from build123d import *

# Parameters (mm, degrees)
BOSS_EXTRUDE1_DEPTH      = 100
BOSS_EXTRUDE1_DEPTH_BACK = 12.5
SKETCH1_W                = 25
SKETCH1_H                = 20
SKETCH2_W                = 15
SKETCH2_H                = 10
CUT_EXTRUDE1_DEPTH       = 103.74361294
CUT_EXTRUDE2_DEPTH       = 103.74361294


with BuildPart() as part:
    # Sketch1 → Boss-Extrude1 (new, two sides: drawn at the far end of the back side and taken through both)
    with BuildSketch(Plane(origin=(0, 0, 0), x_dir=(1, 0, 0), z_dir=(0, 1, 0)).offset(-BOSS_EXTRUDE1_DEPTH_BACK)):
        Rectangle(SKETCH1_W, SKETCH1_H)
    extrude(amount=BOSS_EXTRUDE1_DEPTH + BOSS_EXTRUDE1_DEPTH_BACK)

    # Sketch2 → Cut-Extrude1 (cut, through all)
    with BuildSketch(Plane.XY.offset(10)):
        with Locations((0, 91.5)):
            Rectangle(SKETCH2_W, SKETCH2_H)
    extrude(amount=-CUT_EXTRUDE1_DEPTH, mode=Mode.SUBTRACT)

    # Sketch3 → Cut-Extrude2 (cut, through all)
    with BuildSketch(Plane.XY.offset(10)):
        with BuildLine():
            Line((-3.5, -2.5), (3.5, -2.5))
            ThreePointArc((3.5, -2.5), (7.035533906, -1.035533906), (8.5, 2.5))
            Line((8.5, 2.5), (8.5, 70))
            ThreePointArc((8.5, 70), (7.035533906, 73.535533906), (3.5, 75))
            Line((3.5, 75), (-3.5, 75))
            ThreePointArc((-3.5, 75), (-7.035533906, 73.535533906), (-8.5, 70))
            Line((-8.5, 70), (-8.5, 2.5))
            ThreePointArc((-8.5, 2.5), (-7.035533906, -1.035533906), (-3.5, -2.5))
        make_face()
    extrude(amount=-CUT_EXTRUDE2_DEPTH, mode=Mode.SUBTRACT)


solid = part.part
Work out the finished part from the listing and answer in its coordinate system (mm). A direction names the side the tool comes from. Round coordinates to 2 decimals unless told otherwise and drop trailing zeros. Write each loop counter-clockwise with the first axis right and the second up, starting at its lowest first coordinate (ties: lowest second). Pieces come first, ordered by that corner, then holes.
1) A cutting plane is placed at A-A (y = 16). Give the vertices of the cut face in (x, z).
2) Straight lines are drawn through the part: line 1 (Y direction, x = 2, z = -9); line 2 (X direction, y = 6.5, z = 8.75); line 3 (Y direction, x = -6, z = 1.5). For each, find the intervals that lie inside material, in ascending order.
3) A cutting plane is placed at C-C (z = 5.75). Give the vertices of the cut face in (x, y).
4) A cutting plane is placed at D-D (y = 91). Give the vertices of the cut face in (x, z).
5) A tool of negligible diameter and unlimited length cuts with its end or side. For faces 4 (the flat face through (7.5, 91, 0)), 5 (the flat face through (-12.5, 43, 0)), from which of +Z, -Z, +X, -X, +Y, -Y can it reach the whole face along a straight path? Write none if from no direction.
6) The mould has two halves that part along Y. Classify faces 1 (the flat face through (0, -12.5, 0)), 2 (the flat face through (-9, 43, -10)), 3 (the flat face through (8.5, 36, 0)): pulls with the +Y half, pulls with the -Y half, needs draft (parallel to the pull), parting line crosses it, or undercut.
7) A cutting plane is placed at B-B (x = 2.5). Give the vertices of the cut face in (y, z), plus the area to 3 significant figures.
Completed:
1. outline: (-12.5, -10) - (-8.5, -10) - (-8.5, 10) - (-12.5, 10) - close; (8.5, -10) - (12.5, -10) - (12.5, 10) - (8.5, 10) - close
2. line 1: y = -12.5 to -2.5, 75 to 86.5, 96.5 to 100
2. line 2: x = -12.5 to -8.5, 8.5 to 12.5
2. line 3: y = -12.5 to -1.83, 74.33 to 86.5, 96.5 to 100
3. outline: (-12.5, -12.5) - (12.5, -12.5) - (12.5, 100) - (-12.5, 100) - close; hole (-8.5, 2.5) arc R5 ccw to (-3.5, -2.5) - (3.5, -2.5) arc R5 ccw to (8.5, 2.5) - (8.5, 70) arc R5 ccw to (3.5, 75) - (-3.5, 75) arc R5 ccw to (-8.5, 70) - close; hole (-7.5, 86.5) - (7.5, 86.5) - (7.5, 96.5) - (-7.5, 96.5) - close
4. outline: (-12.5, -10) - (-7.5, -10) - (-7.5, 10) - (-12.5, 10) - close; (7.5, -10) - (12.5, -10) - (12.5, 10) - (7.5, 10) - close
5. face 4: +Z, -Z
5. face 5: +Z, -Z, -X, +Y, -Y
6. face 1: pulls with the -Y half
6. face 2: needs draft
6. face 3: undercut
7. outline: (-12.5, -10) - (-2.5, -10) - (-2.5, 10) - (-12.5, 10) - close; (75, -10) - (86.5, -10) - (86.5, 10) - (75, 10) - close; (96.5, -10) - (100, -10) - (100, 10) - (96.5, 10) - close
7. area: 500 mm2
